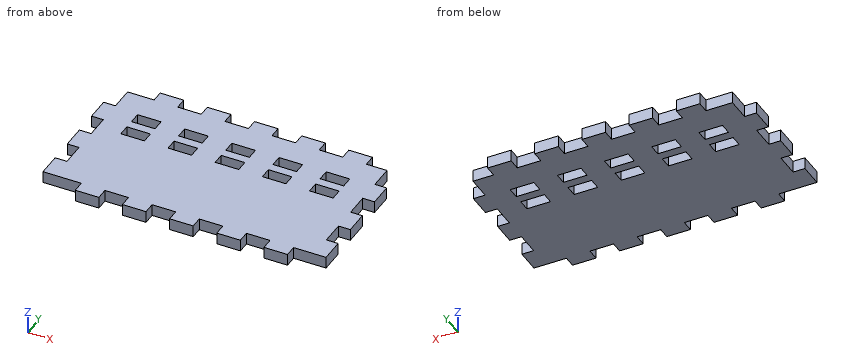
```python
from build123d import *

# Parameters (mm, degrees)
SKETCH1_W               = 279.4
SKETCH1_H               = 152.4
BOSS_EXTRUDE1_DEPTH     = 12.7
SKETCH2_W               = 25.4
SKETCH2_H               = 12.7
BOSS_EXTRUDE2_DEPTH     = 12.7
LPATTERN1_COUNT         = 5
LPATTERN1_PITCH         = 50.8
MIRROR1_COPY_1_SKETCH_W = 25.4
MIRROR1_COPY_1_SKETCH_H = 12.7
MIRROR1_COPY_1_DEPTH    = 12.7
MIRROR1_COPY_2_SKETCH_W = 25.4
MIRROR1_COPY_2_SKETCH_H = 12.7
MIRROR1_COPY_2_DEPTH    = 12.7
MIRROR1_COPY_3_SKETCH_W = 25.4
MIRROR1_COPY_3_SKETCH_H = 12.7
MIRROR1_COPY_3_DEPTH    = 12.7
MIRROR1_COPY_4_SKETCH_W = 25.4
MIRROR1_COPY_4_SKETCH_H = 12.7
MIRROR1_COPY_4_DEPTH    = 12.7
SKETCH3_W               = 12.7
SKETCH3_H               = 25.4
BOSS_EXTRUDE3_DEPTH     = 12.7
LPATTERN2_COUNT         = 3
LPATTERN2_PITCH         = 50.8
MIRROR2_COPY_1_SKETCH_W = 12.7
MIRROR2_COPY_1_SKETCH_H = 25.4
MIRROR2_COPY_1_DEPTH    = 12.7
MIRROR2_COPY_2_SKETCH_W = 12.7
MIRROR2_COPY_2_SKETCH_H = 25.4
MIRROR2_COPY_2_DEPTH    = 12.7
SKETCH4_W               = 25.4
SKETCH4_H               = 12.7
CUT_EXTRUDE1_DEPTH      = 13.7
LPATTERN3_COUNT         = 5
LPATTERN3_PITCH         = 50.8


with BuildPart() as part:
    # Sketch1 → Boss-Extrude1 (new body)
    with BuildSketch(Plane.XY):
        Rectangle(SKETCH1_W, SKETCH1_H)
    extrude(amount=BOSS_EXTRUDE1_DEPTH)

    # Sketch2 → Boss-Extrude2 (add)
    with BuildSketch(Plane.XZ.offset(76.2)):
        with Locations((-98.425, 6.35)):
            Rectangle(SKETCH2_W, SKETCH2_H)
    boss_extrude2 = extrude(amount=BOSS_EXTRUDE2_DEPTH)

    # LPattern1: Boss-Extrude2 ×5
    with Locations(*[(i * LPATTERN1_PITCH, 0, 0) for i in range(1, LPATTERN1_COUNT)]):
        add(boss_extrude2)

    # Mirror1: Boss-Extrude2 across plane
    add(boss_extrude2.mirror(Plane.ZX))

    # Mirror1 copy 1 sketch → Mirror1 copy 1 (add)
    with BuildSketch(Plane(origin=(50.8, 76.2, 0), x_dir=(1, 0, 0), z_dir=(0, 1, 0))):
        with Locations((-98.425, -6.35)):
            Rectangle(MIRROR1_COPY_1_SKETCH_W, MIRROR1_COPY_1_SKETCH_H)
    extrude(amount=MIRROR1_COPY_1_DEPTH)

    # Mirror1 copy 2 sketch → Mirror1 copy 2 (add)
    with BuildSketch(Plane(origin=(101.6, 76.2, 0), x_dir=(1, 0, 0), z_dir=(0, 1, 0))):
        with Locations((-98.425, -6.35)):
            Rectangle(MIRROR1_COPY_2_SKETCH_W, MIRROR1_COPY_2_SKETCH_H)
    extrude(amount=MIRROR1_COPY_2_DEPTH)

    # Mirror1 copy 3 sketch → Mirror1 copy 3 (add)
    with BuildSketch(Plane(origin=(152.4, 76.2, 0), x_dir=(1, 0, 0), z_dir=(0, 1, 0))):
        with Locations((-98.425, -6.35)):
            Rectangle(MIRROR1_COPY_3_SKETCH_W, MIRROR1_COPY_3_SKETCH_H)
    extrude(amount=MIRROR1_COPY_3_DEPTH)

    # Mirror1 copy 4 sketch → Mirror1 copy 4 (add)
    with BuildSketch(Plane(origin=(203.2, 76.2, 0), x_dir=(1, 0, 0), z_dir=(0, 1, 0))):
        with Locations((-98.425, -6.35)):
            Rectangle(MIRROR1_COPY_4_SKETCH_W, MIRROR1_COPY_4_SKETCH_H)
    extrude(amount=MIRROR1_COPY_4_DEPTH)

    # Sketch3 → Boss-Extrude3 (add)
    with BuildSketch(Plane(origin=(139.7, 0, 0), x_dir=(0, 0, -1), z_dir=(1, 0, 0))):
        with Locations((-6.35, -63.5)):
            Rectangle(SKETCH3_W, SKETCH3_H)
    boss_extrude3 = extrude(amount=BOSS_EXTRUDE3_DEPTH)

    # LPattern2: Boss-Extrude3 ×3
    with Locations(*[(0, i * LPATTERN2_PITCH, 0) for i in range(1, LPATTERN2_COUNT)]):
        add(boss_extrude3)

    # Mirror2: Boss-Extrude3 across plane
    add(boss_extrude3.mirror(Plane(origin=(0, 0, 0), x_dir=(0, 0, 1), z_dir=(1, 0, 0))))

    # Mirror2 copy 1 sketch → Mirror2 copy 1 (add)
    with BuildSketch(Plane(origin=(-139.7, 50.8, 0), x_dir=(0, 0, -1), z_dir=(-1, 0, 0))):
        with Locations((-6.35, 63.5)):
            Rectangle(MIRROR2_COPY_1_SKETCH_W, MIRROR2_COPY_1_SKETCH_H)
    extrude(amount=MIRROR2_COPY_1_DEPTH)

    # Mirror2 copy 2 sketch → Mirror2 copy 2 (add)
    with BuildSketch(Plane(origin=(-139.7, 101.6, 0), x_dir=(0, 0, -1), z_dir=(-1, 0, 0))):
        with Locations((-6.35, 63.5)):
            Rectangle(MIRROR2_COPY_2_SKETCH_W, MIRROR2_COPY_2_SKETCH_H)
    extrude(amount=MIRROR2_COPY_2_DEPTH)

    # Sketch4 → Cut-Extrude1 (cut, through all)
    with BuildSketch(Plane.XY.offset(12.7)):
        with Locations((-101.6, 19.05)):
            Rectangle(SKETCH4_W, SKETCH4_H)
        with Locations((-101.6, 41.275)):
            Rectangle(SKETCH4_W, SKETCH4_H)
    cut_extrude1 = extrude(amount=-CUT_EXTRUDE1_DEPTH, mode=Mode.SUBTRACT)

    # LPattern3: Cut-Extrude1 ×5
    with Locations(*[(i * LPATTERN3_PITCH, 0, 0) for i in range(1, LPATTERN3_COUNT)]):
        add(cut_extrude1, mode=Mode.SUBTRACT)


solid = part.part
```
Could you check a few things on this model? Use its own coordinates, in mm. Give positions to 0.01 mm unless a question says otherwise; leave off trailing zeros. Order: outer loops, then holes, each group sorted by start corner. A loop starts at its lowest first (then second) coordinate and runs counter-clockwise, first axis right, second up.
Q1. Suppose I cut it at C-C, the plane y = 9. Write out the boundary of the cut face in (x, z).
Q2. If I drill on line 1 along Y through (x, z) = (4, 6.25) (3 decimals); line 2 along Y through (x, z) = (-12.5, 1.25) (3 decimals); line 3 along X through (y, z) = (-79, 1.75) (3 decimals), over which ranges is the centre line in solid material (lowest first)?
Q3. Suppose I cut it at B-B, the plane z = 5. Count the separate pieces of the cut face and the enclosed holes in it, and give its area (3 significant figures).
Q4. Suppose I cut it at A-A, the plane y = 42.5. Write out the boundary of the cut face in (x, z), and give its area (3 significant figures).
Q5. I'm going to push flat-ended pins straight in: P1, Ø6.5, axis at y = -85, z = 4, coming from the -X side (3 decimals); P2, Ø1.5, axis at x = 74, z = 2.5, coming from the -Y side; P3, Ø6, axis at x = -114.5, z = 7, coming from the +Y side. Where does each tip first touch, or does it pass through?
Q6. Suppose I cut it at D-D, the plane x = 75.5. Write out the boundary of the cut face in (y, z).
Solution:
1. outline: (-139.7, 0) - (139.7, 0) - (139.7, 12.7) - (-139.7, 12.7) - close
2. line 1: y = -88.9 to 12.7, 25.4 to 34.925, 47.625 to 88.9
2. line 2: y = -76.2 to 12.7, 25.4 to 34.925, 47.625 to 76.2
2. line 3: x = -111.125 to -85.725, -60.325 to -34.925, -9.525 to 15.875, 41.275 to 66.675, 92.075 to 117.475
3. separate pieces: 1
3. enclosed holes: 10
3. area: 44,500 mm2
4. outline: (-152.4, 0) - (-114.3, 0) - (-114.3, 12.7) - (-152.4, 12.7) - close; (-88.9, 0) - (-63.5, 0) - (-63.5, 12.7) - (-88.9, 12.7) - close; (-38.1, 0) - (-12.7, 0) - (-12.7, 12.7) - (-38.1, 12.7) - close; (12.7, 0) - (38.1, 0) - (38.1, 12.7) - (12.7, 12.7) - close; (63.5, 0) - (88.9, 0) - (88.9, 12.7) - (63.5, 12.7) - close; (114.3, 0) - (152.4, 0) - (152.4, 12.7) - (114.3, 12.7) - close
4. area: 2,260 mm2
5. P1: stops at x = -111.125
5. P2: stops at y = -76.2
5. P3: stops at y = 76.2
6. outline: (-76.2, 0) - (76.2, 0) - (76.2, 12.7) - (-76.2, 12.7) - close
